Input: part model. Units: mm. Frame: model coordinates. A direction names the side the tool comes from. Round coordinates to 2 decimals unless told otherwise and drop trailing zeros. Loops run counter-clockwise (first coordinate to the right, second up) from the corner with the lowest first, then second, coordinate; pieces in that order, holes last. Notation, with made-up numbers: (39, 22.5) -> (85, 22.5) arc R24 ccw to (85, 59.5) -> close; hole circle Ø4 at (58, -15.75). An arc over 180 degrees is marked (long way). Answer as a JSON object with one key per item and string values.
```python
from build123d import *

# Parameters (mm, degrees)
SKETCH_R     = 12
PAD_DEPTH    = 16
POCKET_DEPTH = 8
FILLET_R     = 0.6
SKETCH002_R  = 8
PAD001_DEPTH = 2
SKETCH003_R  = 6
PAD002_DEPTH = 55


with BuildPart() as part:
    # Sketch → Pad (new body)
    with BuildSketch(Plane.XY):
        Circle(SKETCH_R)
    extrude(amount=PAD_DEPTH)

    # Sketch001 (on Face2 of Pad) → Pocket (cut)
    with BuildSketch(Plane(origin=(0, 0, 0), x_dir=(1, 0, 0), z_dir=(0, 0, -1))):
        Polygon((0, -8.082904), (7, -4.041452), (7, 4.041452), (0, 8.082904), (-7, 4.041452), (-7, -4.041452), align=None)
    extrude(amount=-POCKET_DEPTH, mode=Mode.SUBTRACT)

    # Fillet
    fillet_edges = [part.edges().sort_by_distance(p)[0] for p in [
        (-12, 0, 0),
    ]]
    fillet(fillet_edges, radius=FILLET_R)

    # Sketch002 (on Face3 of Fillet) → Pad001 (join)
    with BuildSketch(Plane.XY.offset(16)):
        Circle(SKETCH002_R)
    extrude(amount=PAD001_DEPTH)

    # Sketch003 (on Face12 of Pad001) → Pad002 (join)
    with BuildSketch(Plane.XY.offset(18)):
        Circle(SKETCH003_R)
    extrude(amount=PAD002_DEPTH)


solid = part.part
```
1) Reachability of faces 1 (the face through (-6, 0, 45)), 2 (the face through (-7, 0, 4)), 3 (the face through (0, 0, 73)) from +Z, -Z, +X, -X, +Y, -Y: full face, straight path, thin tool, end or side. Return the list, or none.
Output:
{"face 1": "+Z", "face 2": "-Z", "face 3": "+Z, +X, -X, +Y, -Y"}
2) Ray query, probe 1 along Z at (x, y) = (3.25, -9.5); probe 2 along Y at (x, z) = (0.5, 7); probe 3 along Z at (x, y) = (0.75, 2). Return the intervals inside material, ascending.
Output:
{"probe 1": "z = 0 to 16", "probe 2": "y = -11.99 to -7.79, 7.79 to 11.99", "probe 3": "z = 8 to 73"}
3) Section C-C, the plane z = 58.5. Output: boundary loops of the cut face in (x, y), plus the area to 3 significant figures.
Output:
{"outline": "circle Ø12 at (0, 0)", "area": "113 mm^2"}
4) Section A-A, the plane y = 0. Output: boundary loops of the cut face in (x, z).
Output:
{"outline": "(-12, 0.6) arc R0.6 ccw to (-11.4, 0) -> (-7, 0) -> (-7, 8) -> (7, 8) -> (7, 0) -> (11.4, 0) arc R0.6 ccw to (12, 0.6) -> (12, 16) -> (8, 16) -> (8, 18) -> (6, 18) -> (6, 73) -> (-6, 73) -> (-6, 18) -> (-8, 18) -> (-8, 16) -> (-12, 16) -> close"}
5) Draft query along Y for faces 4 (the face through (-3.45, -6.09, 3.94)), 5 (the face through (-11.99, 0.53, 8.19)), 6 (the face through (-2, 6, 18)), 7 (the face through (3.549, -6.034, 3.944)). Return one class per face: +Y half, -Y half, draft (parallel to the pull), parting line (faces both ways), or undercut.
Output:
{"face 4": "undercut", "face 5": "parting line", "face 6": "draft", "face 7": "undercut"}
6) Section B-B, the plane z = 9. Output: boundary loops of the cut face in (x, y).
Output:
{"outline": "circle Ø24 at (0, 0)"}
7) Contact query for flat-ended pins moving along their axis: P1, Ø3, axis at y = -1, z = 24, coming from the -X side; P2, Ø8, axis at y = 7.5, z = 24, coming from the +X side; P3, Ø5, axis at y = 4.5, z = 33, coming from the +X side. Output: stop coordinate, or through.
Output:
{"P1": "stops at x = -6", "P2": "stops at x = 4.87", "P3": "stops at x = 5.66"}
